Read the model definition and answer for the solid it produces. Units are mm, in the model's axes. A direction names the side the tool comes from. Round coordinates to 2 decimals unless told otherwise and drop trailing zeros. Order: outer loops, then holes, each group sorted by start corner. A loop starts at its lowest first (then second) coordinate and runs counter-clockwise, first axis right, second up. Notation, with made-up numbers: (78.5, 25.5) -> (124.5, 25.5) arc R21 cw to (124.5, 32.5) -> close; hole circle Ø10 at (31, 38.25). An arc over 180 degrees is marked (long way). Use a Markdown table: item, result. Add a question column.
1. Section B-B, the plane y = 6.35 is taken. Give the vertices of the cut face in (x, z) (3 decimals).
2. Section A-A, the plane x = 8.25 is taken. Give the vertices of the cut face in (y, z) (3 decimals).
3. Consider L1, parallel to Z at x = 7.5, y = 3; L2, parallel to X at y = 6.5, z = 22.75; L3, parallel to X at y = 15, z = 4. Determine where each line is inside the solid, lowest interval first. Write a range as [from, to].
4. Given pin 1 (5 mm diameter, centred on y = 7.5, z = 8, fed in from +X), flat-ended and moving along its own axis, determine where the tip first touches the part or whether it passes through.
5. Section D-D, the plane z = 7.75 is taken. Give the vertices of the cut face in (x, y), then the cut area to 3 significant figures.
6. Section C-C, the plane z = 11.5 is taken. Give the vertices of the cut face in (x, y).
7. For faces 5 (the face through (3.83, 15.751, 0.724)), 6 (the face through (9.569, 10.182, 4.096)), determine the directions among +Z, -Z, +X, -X, +Y, -Y from which every point of the face is accessible in a straight line to the end or side of a thin tool.
8. The mould has two halves that part along Z. Classify faces 1 (the face through (0.323, 14.067, 12.558)), 2 (the face through (11.936, 9.22, 0.724)), 3 (the face through (9.569, 2.518, 21.304)), 4 (the face through (6.35, 4, 19)): +Z half, -Z half, draft (parallel to the pull), parting line (faces both ways), or undercut.
```python
from build123d import *

# Parameters (mm, degrees)
BOSS_EXTRUDE1_DEPTH = 25.4
SKETCH4_R           = 2.159
CUT_EXTRUDE1_DEPTH  = 34.76004538
CUT_EXTRUDE2_DEPTH  = 6.35
FILLET1_R           = 2.54


with BuildPart() as part:
    # Sketch3 → Boss-Extrude1 (new body)
    with BuildSketch(Plane.XY):
        Polygon((0, 14.224), (6.35, 18.25625), (12.7, 18.25625), (12.7, 0), (0, 0), align=None)
    extrude(amount=BOSS_EXTRUDE1_DEPTH)

    # Sketch4 → Cut-Extrude1 (cut, through all)
    with BuildSketch(Plane.ZY):
        with Locations((6.35, 6.35)):
            Circle(SKETCH4_R)
        with Locations((19.05, 6.35)):
            Circle(SKETCH4_R)
    extrude(amount=-CUT_EXTRUDE1_DEPTH, mode=Mode.SUBTRACT)

    # Sketch6 → Cut-Extrude2 (cut)
    with BuildSketch(Plane(origin=(12.7, 0, 0), x_dir=(0, 0, -1), z_dir=(1, 0, 0))):
        Polygon((-14.605, 8.916321947), (-19.05, 11.482643893), (-23.495, 8.916321947), (-23.495, 3.783678053), (-19.05, 1.217356107), (-14.605, 3.783678053), align=None)
        Polygon((-1.905, 3.783678053), (-1.905, 8.916321947), (-6.35, 11.482643893), (-10.795, 8.916321947), (-10.795, 3.783678053), (-6.35, 1.217356107), align=None)
    extrude(amount=-CUT_EXTRUDE2_DEPTH, mode=Mode.SUBTRACT)

    # Fillet1
    # the kernel refuses this fillet: 2.54 mm, written as the material it takes off along each edge
    with BuildSketch(Plane(origin=(2.54, 2.54, 2.54), x_dir=(0, 0, -1), z_dir=(-1, 0, 0))) as fillet1_piece_1_section:
        Polygon((0, 0), (FILLET1_R, 0), (FILLET1_R, FILLET1_R), (0, FILLET1_R), align=None)
    fillet1_piece_1 = extrude(amount=FILLET1_R, mode=Mode.PRIVATE)
    fillet1_piece_1 = fillet1_piece_1 - Plane(origin=(2.54, 2.54, 2.54), x_dir=(0, 0.7071067811865475, 0.7071067811865475), z_dir=(-1, 0, 0)) * Sphere(FILLET1_R, mode=Mode.PRIVATE)
    add(fillet1_piece_1, mode=Mode.SUBTRACT)
    with BuildSketch(Plane(origin=(2.54, 2.54, 22.86), x_dir=(0, 0, 1), z_dir=(-1, 0, 0))) as fillet1_piece_2_section:
        Polygon((0, 0), (FILLET1_R, 0), (FILLET1_R, -FILLET1_R), (0, -FILLET1_R), align=None)
    fillet1_piece_2 = extrude(amount=FILLET1_R, mode=Mode.PRIVATE)
    fillet1_piece_2 = fillet1_piece_2 - Plane(origin=(2.54, 2.54, 22.86), x_dir=(0, 0.7071067811865475, -0.7071067811865475), z_dir=(-1, 0, 0)) * Sphere(FILLET1_R, mode=Mode.PRIVATE)
    add(fillet1_piece_2, mode=Mode.SUBTRACT)
    with BuildSketch(Plane(origin=(10.16, 2.54, 2.54), x_dir=(0, 0, -1), z_dir=(1, 0, 0))) as fillet1_piece_3_section:
        Polygon((0, 0), (FILLET1_R, 0), (FILLET1_R, -FILLET1_R), (0, -FILLET1_R), align=None)
    fillet1_piece_3 = extrude(amount=FILLET1_R, mode=Mode.PRIVATE)
    fillet1_piece_3 = fillet1_piece_3 - Plane(origin=(10.16, 2.54, 2.54), x_dir=(0, 0.7071067811865475, 0.7071067811865475), z_dir=(1, 0, 0)) * Sphere(FILLET1_R, mode=Mode.PRIVATE)
    add(fillet1_piece_3, mode=Mode.SUBTRACT)
    with BuildSketch(Plane(origin=(10.16, 2.54, 22.86), x_dir=(0, 0, 1), z_dir=(1, 0, 0))) as fillet1_piece_4_section:
        Polygon((0, 0), (FILLET1_R, 0), (FILLET1_R, FILLET1_R), (0, FILLET1_R), align=None)
    fillet1_piece_4 = extrude(amount=FILLET1_R, mode=Mode.PRIVATE)
    fillet1_piece_4 = fillet1_piece_4 - Plane(origin=(10.16, 2.54, 22.86), x_dir=(0, 0.7071067811865475, -0.7071067811865475), z_dir=(1, 0, 0)) * Sphere(FILLET1_R, mode=Mode.PRIVATE)
    add(fillet1_piece_4, mode=Mode.SUBTRACT)
    with BuildSketch(Plane(origin=(10.16, 15.71625, 2.54), x_dir=(0, 1, 0), z_dir=(1, 0, 0))) as fillet1_piece_5_section:
        Polygon((0, 0), (FILLET1_R, 0), (FILLET1_R, -FILLET1_R), (0, -FILLET1_R), align=None)
    fillet1_piece_5 = extrude(amount=FILLET1_R, mode=Mode.PRIVATE)
    fillet1_piece_5 = fillet1_piece_5 - Plane(origin=(10.16, 15.71625, 2.54), x_dir=(0, -0.7071067811865475, 0.7071067811865475), z_dir=(1, 0, 0)) * Sphere(FILLET1_R, mode=Mode.PRIVATE)
    add(fillet1_piece_5, mode=Mode.SUBTRACT)
    with BuildSketch(Plane(origin=(10.16, 15.71625, 22.86), x_dir=(0, 1, 0), z_dir=(1, 0, 0))) as fillet1_piece_6_section:
        Polygon((0, 0), (FILLET1_R, 0), (FILLET1_R, FILLET1_R), (0, FILLET1_R), align=None)
    fillet1_piece_6 = extrude(amount=FILLET1_R, mode=Mode.PRIVATE)
    fillet1_piece_6 = fillet1_piece_6 - Plane(origin=(10.16, 15.71625, 22.86), x_dir=(0, -0.7071067811865475, -0.7071067811865475), z_dir=(1, 0, 0)) * Sphere(FILLET1_R, mode=Mode.PRIVATE)
    add(fillet1_piece_6, mode=Mode.SUBTRACT)
    with BuildSketch(Plane(origin=(7.088311936, 15.71625, 2.54), x_dir=(-0.5360558854014316, 0.8441824966951682, 0), z_dir=(0, 0, -1))) as fillet1_piece_7_section:
        Polygon((0, 0), (FILLET1_R, 0), (FILLET1_R, FILLET1_R * 0.290673990433), (FILLET1_R * 0.844182496695, FILLET1_R * 0.536055885401), align=None)
    fillet1_piece_7 = extrude(amount=FILLET1_R, mode=Mode.PRIVATE)
    fillet1_piece_7 = fillet1_piece_7 - Plane(origin=(7.088311936, 15.71625, 2.54), x_dir=(0.2791213923231542, -0.9602558244278364, 0), z_dir=(0, 0, -1)) * Sphere(FILLET1_R, mode=Mode.PRIVATE)
    add(fillet1_piece_7, mode=Mode.SUBTRACT)
    with BuildSketch(Plane(origin=(7.088311936, 15.71625, 22.86), x_dir=(-0.5360558854014316, 0.8441824966951682, 0), z_dir=(0, 0, 1))) as fillet1_piece_8_section:
        Polygon((0, 0), (FILLET1_R, 0), (FILLET1_R, -FILLET1_R * 0.290673990433), (FILLET1_R * 0.844182496695, -FILLET1_R * 0.536055885401), align=None)
    fillet1_piece_8 = extrude(amount=FILLET1_R, mode=Mode.PRIVATE)
    fillet1_piece_8 = fillet1_piece_8 - Plane(origin=(7.088311936, 15.71625, 22.86), x_dir=(0.2791213923231542, -0.9602558244278364, 0), z_dir=(0, 0, 1)) * Sphere(FILLET1_R, mode=Mode.PRIVATE)
    add(fillet1_piece_8, mode=Mode.SUBTRACT)
    with BuildSketch(Plane(origin=(2.54, 12.828071921, 22.86), x_dir=(-0.5360558854014316, 0.8441824966951682, 0), z_dir=(0, 0, 1))) as fillet1_piece_9_section:
        Polygon((0, 0), (FILLET1_R, 0), (FILLET1_R, FILLET1_R * 0.549577983925), (FILLET1_R * 0.536055885401, FILLET1_R * 0.844182496695), align=None)
    fillet1_piece_9 = extrude(amount=FILLET1_R, mode=Mode.PRIVATE)
    fillet1_piece_9 = fillet1_piece_9 - Plane(origin=(2.54, 12.828071921, 22.86), x_dir=(0.8763720344127349, -0.4816347758408693, 0), z_dir=(0, 0, 1)) * Sphere(FILLET1_R, mode=Mode.PRIVATE)
    add(fillet1_piece_9, mode=Mode.SUBTRACT)
    with BuildSketch(Plane(origin=(2.54, 12.828071921, 2.54), x_dir=(-0.5360558854014316, 0.8441824966951682, 0), z_dir=(0, 0, -1))) as fillet1_piece_10_section:
        Polygon((0, 0), (FILLET1_R, 0), (FILLET1_R, -FILLET1_R * 0.549577983925), (FILLET1_R * 0.536055885401, -FILLET1_R * 0.844182496695), align=None)
    fillet1_piece_10 = extrude(amount=FILLET1_R, mode=Mode.PRIVATE)
    fillet1_piece_10 = fillet1_piece_10 - Plane(origin=(2.54, 12.828071921, 2.54), x_dir=(0.8763720344127349, -0.4816347758408693, 0), z_dir=(0, 0, -1)) * Sphere(FILLET1_R, mode=Mode.PRIVATE)
    add(fillet1_piece_10, mode=Mode.SUBTRACT)
    with BuildSketch(Plane(origin=(0, 0, 2.54), x_dir=(0, 1, 0), z_dir=(0, 0, 1)), Plane(origin=(12.7, 0, 2.54), x_dir=(-1, 0, 0), z_dir=(0, 0, 1))) as fillet1_piece_11:
        with BuildLine():
            CenterArc((FILLET1_R, -FILLET1_R), FILLET1_R, 90, 90)
            Line((0, -FILLET1_R), (0, 0))
            Line((0, 0), (FILLET1_R, 0))
        make_face()
    extrude(amount=20.32, mode=Mode.SUBTRACT)
    with BuildSketch(Plane(origin=(12.7, 18.25625, 2.54), x_dir=(-1, 0, 0), z_dir=(0, 0, 1))) as fillet1_piece_12:
        with BuildLine():
            CenterArc((FILLET1_R, FILLET1_R), FILLET1_R, 180, 90)
            Line((0, FILLET1_R), (0, 0))
            Line((0, 0), (FILLET1_R, 0))
        make_face()
    extrude(amount=20.32, mode=Mode.SUBTRACT)
    with BuildSketch(Plane(origin=(6.35, 18.25625, 2.54), x_dir=(-0.8441824966951671, -0.536055885401433, 0), z_dir=(0, 0, 1))) as fillet1_piece_13:
        with BuildLine():
            CenterArc((FILLET1_R * 0.290673990433, FILLET1_R), FILLET1_R, 237.58445267, 32.41554733)
            Line((-FILLET1_R * 0.245381894968, FILLET1_R * 0.155817503305), (0, 0))
            Line((0, 0), (FILLET1_R * 0.290673990433, 0))
        make_face()
    extrude(amount=20.32, mode=Mode.SUBTRACT)
    with BuildSketch(Plane(origin=(1.178418051, 14.972295462, 25.4), x_dir=(0, 0, -1), z_dir=(0.844182496695168, 0.5360558854014315, 0))) as fillet1_piece_14:
        with BuildLine():
            CenterArc((FILLET1_R, -FILLET1_R), FILLET1_R, 90, 90)
            Line((0, -FILLET1_R), (0, 0))
            Line((0, 0), (FILLET1_R, 0))
        make_face()
    extrude(amount=5.387830183, mode=Mode.SUBTRACT)
    with BuildSketch(Plane(origin=(7.088311936, 18.25625, 25.4), x_dir=(0, 0, -1), z_dir=(1, 0, 0))) as fillet1_piece_15:
        with BuildLine():
            CenterArc((FILLET1_R, -FILLET1_R), FILLET1_R, 90, 90)
            Line((0, -FILLET1_R), (0, 0))
            Line((0, 0), (FILLET1_R, 0))
        make_face()
    extrude(amount=3.071688064, mode=Mode.SUBTRACT)
    with BuildSketch(Plane(origin=(12.7, 15.71625, 25.4), x_dir=(-1, 0, 0), z_dir=(0, -1, 0))) as fillet1_piece_16:
        with BuildLine():
            CenterArc((FILLET1_R, FILLET1_R), FILLET1_R, 180, 90)
            Line((0, FILLET1_R), (0, 0))
            Line((0, 0), (FILLET1_R, 0))
        make_face()
    extrude(amount=13.17625, mode=Mode.SUBTRACT)
    with BuildSketch(Plane(origin=(10.16, 0, 25.4), x_dir=(0, 1, 0), z_dir=(-1, 0, 0))) as fillet1_piece_17:
        with BuildLine():
            CenterArc((FILLET1_R, FILLET1_R), FILLET1_R, 180, 90)
            Line((0, FILLET1_R), (0, 0))
            Line((0, 0), (FILLET1_R, 0))
        make_face()
    extrude(amount=7.62, mode=Mode.SUBTRACT)
    with BuildSketch(Plane(origin=(0, 2.54, 25.4), x_dir=(0, 0, -1), z_dir=(0, 1, 0))) as fillet1_piece_18:
        with BuildLine():
            CenterArc((FILLET1_R, -FILLET1_R), FILLET1_R, 90, 90)
            Line((0, -FILLET1_R), (0, 0))
            Line((0, 0), (FILLET1_R, 0))
        make_face()
    extrude(amount=10.288071921, mode=Mode.SUBTRACT)
    with BuildSketch(Plane(origin=(10.16, 0, 0), x_dir=(0, 1, 0), z_dir=(-1, 0, 0))) as fillet1_piece_19:
        with BuildLine():
            CenterArc((FILLET1_R, -FILLET1_R), FILLET1_R, 90, 90)
            Line((0, -FILLET1_R), (0, 0))
            Line((0, 0), (FILLET1_R, 0))
        make_face()
    extrude(amount=7.62, mode=Mode.SUBTRACT)
    with BuildSketch(Plane(origin=(12.7, 15.71625, 0), x_dir=(-1, 0, 0), z_dir=(0, -1, 0))) as fillet1_piece_20:
        with BuildLine():
            CenterArc((FILLET1_R, -FILLET1_R), FILLET1_R, 90, 90)
            Line((0, -FILLET1_R), (0, 0))
            Line((0, 0), (FILLET1_R, 0))
        make_face()
    extrude(amount=13.17625, mode=Mode.SUBTRACT)
    with BuildSketch(Plane(origin=(7.088311936, 18.25625, 0), x_dir=(0, 0, 1), z_dir=(1, 0, 0))) as fillet1_piece_21:
        with BuildLine():
            CenterArc((FILLET1_R, FILLET1_R), FILLET1_R, 180, 90)
            Line((0, FILLET1_R), (0, 0))
            Line((0, 0), (FILLET1_R, 0))
        make_face()
    extrude(amount=3.071688064, mode=Mode.SUBTRACT)
    with BuildSketch(Plane(origin=(1.178418051, 14.972295462, 0), x_dir=(0, 0, 1), z_dir=(0.844182496695168, 0.5360558854014315, 0))) as fillet1_piece_22:
        with BuildLine():
            CenterArc((FILLET1_R, FILLET1_R), FILLET1_R, 180, 90)
            Line((0, FILLET1_R), (0, 0))
            Line((0, 0), (FILLET1_R, 0))
        make_face()
    extrude(amount=5.387830183, mode=Mode.SUBTRACT)
    with BuildSketch(Plane(origin=(0, 2.54, 0), x_dir=(0, 0, 1), z_dir=(0, 1, 0))) as fillet1_piece_23:
        with BuildLine():
            CenterArc((FILLET1_R, FILLET1_R), FILLET1_R, 180, 90)
            Line((0, FILLET1_R), (0, 0))
            Line((0, 0), (FILLET1_R, 0))
        make_face()
    extrude(amount=10.288071921, mode=Mode.SUBTRACT)
    with BuildSketch(Plane(origin=(0, 14.224, 2.54), x_dir=(0.844182496695168, 0.5360558854014316, 0), z_dir=(0, 0, 1))) as fillet1_piece_24:
        with BuildLine():
            CenterArc((FILLET1_R * 0.549577983925, -FILLET1_R), FILLET1_R, 90, 57.58445267)
            Line((-FILLET1_R * 0.29460451277, -FILLET1_R * 0.463944114599), (0, 0))
            Line((0, 0), (FILLET1_R * 0.549577983925, 0))
        make_face()
    extrude(amount=20.32, mode=Mode.SUBTRACT)


solid = part.part
```
Verdict:
| question | item | result |
|---|---|---|
| 1 | outline | (0, 2.54) arc R2.54 ccw to (2.54, 0) -> (10.16, 0) arc R2.54 ccw to (12.619, 1.905) -> (6.35, 1.905) -> (6.35, 4.191) -> (0, 4.191) -> close; (0, 8.509) -> (6.35, 8.509) -> (6.35, 10.795) -> (12.7, 10.795) -> (12.7, 14.605) -> (6.35, 14.605) -> (6.35, 16.891) -> (0, 16.891) -> close; (0, 21.209) -> (6.35, 21.209) -> (6.35, 23.495) -> (12.619, 23.495) arc R2.54 ccw to (10.16, 25.4) -> (2.54, 25.4) arc R2.54 ccw to (0, 22.86) -> close |
| 2 | outline | (0, 2.54) arc R2.54 ccw to (2.54, 0) -> (15.716, 0) arc R2.54 ccw to (18.256, 2.54) -> (18.256, 22.86) arc R2.54 ccw to (15.716, 25.4) -> (2.54, 25.4) arc R2.54 ccw to (0, 22.86) -> close; hole (1.217, 6.35) -> (3.784, 1.905) -> (8.916, 1.905) -> (11.483, 6.35) -> (8.916, 10.795) -> (3.784, 10.795) -> close; hole (1.217, 19.05) -> (3.784, 14.605) -> (8.916, 14.605) -> (11.483, 19.05) -> (8.916, 23.495) -> (3.784, 23.495) -> close |
| 3 | L1 | z = [0, 3.26], [9.44, 15.96], [22.14, 25.4] |
| 3 | L2 | x = [0, 6.35] |
| 3 | L3 | x = [1.22, 12.7] |
| 4 | pin 1 | stops at x = 6.35 |
| 5 | outline | (0, 2.54) arc R2.54 ccw to (2.54, 0) -> (10.16, 0) arc R2.54 ccw to (12.65, 2.03) -> (6.35, 2.03) -> (6.35, 4.71) -> (0, 4.71) -> close; (0, 7.99) -> (6.35, 7.99) -> (6.35, 10.67) -> (12.7, 10.67) -> (12.7, 15.72) arc R2.54 ccw to (10.16, 18.26) -> (7.09, 18.26) arc R2.54 ccw to (5.73, 17.86) -> (1.18, 14.97) arc R2.54 ccw to (0, 12.83) -> close |
| 5 | area | 139 mm2 |
| 6 | outline | (0, 2.54) arc R2.54 ccw to (2.54, 0) -> (10.16, 0) arc R2.54 ccw to (12.7, 2.54) -> (12.7, 15.72) arc R2.54 ccw to (10.16, 18.26) -> (7.09, 18.26) arc R2.54 ccw to (5.73, 17.86) -> (1.18, 14.97) arc R2.54 ccw to (0, 12.83) -> close |
| 7 | face 5 | -Z, -X, +Y |
| 7 | face 6 | +X |
| 8 | face 1 | draft |
| 8 | face 2 | -Z half |
| 8 | face 3 | undercut |
| 8 | face 4 | undercut |
